The drawing under review shows one solid part. Ordinate dimensions are in mm from its lowest x, y, z. A direction names the side the tool comes from. Round coordinates to 2 decimals unless told otherwise and drop trailing zeros. Order: outer loops, then holes, each group sorted by start corner. A loop starts at its lowest first (then second) coordinate and runs counter-clockwise, first axis right, second up. Notation, with made-up numbers: M -14.5,30 L 40.5,30 A21 ccw 40.5,52 Z; hole C 17.5,59 d11. An arc over 180 degrees is marked long. Answer as a JSON object with one key per item and string values.
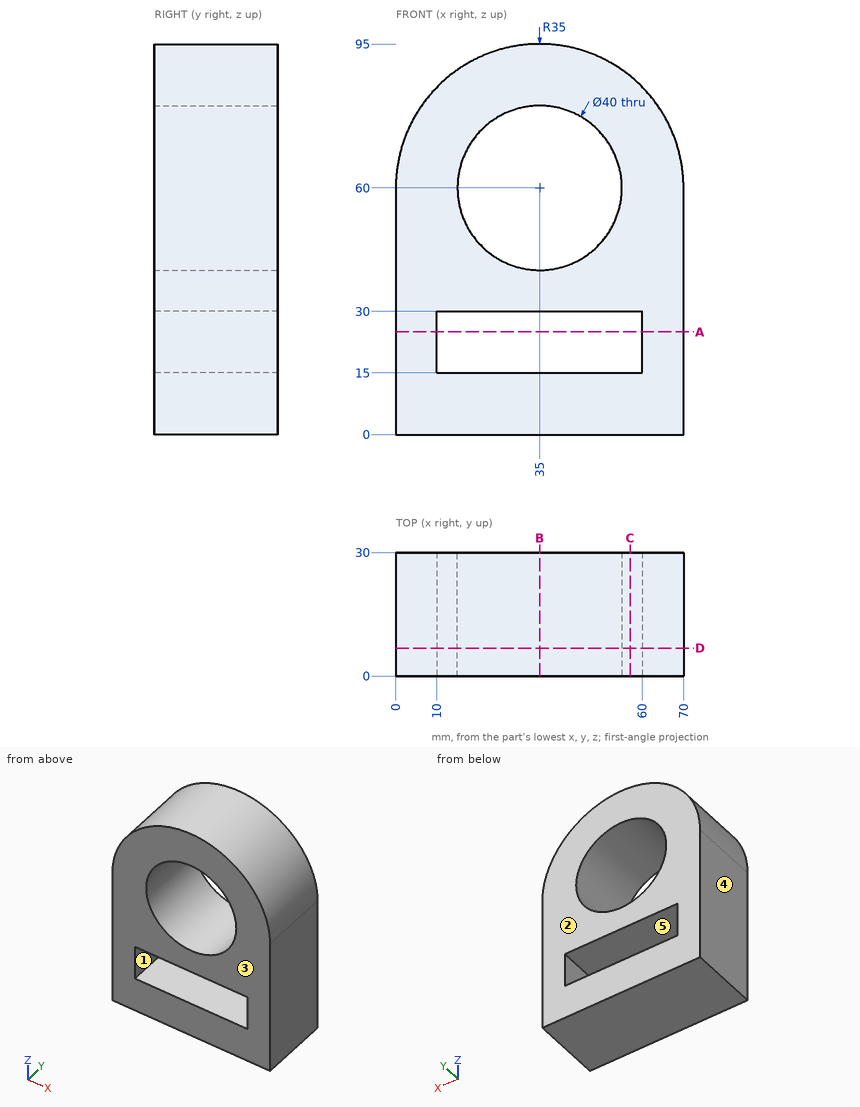
1) For L1, parallel to Z at x = 35, y = 22; L2, parallel to X at y = 21, z = 19; L3, parallel to Z at x = 33.5, y = 16.25, list the stretches that pass through material, from the lowest coordinate up.
Geometry check:
{"L1": "z = 0 to 15, 30 to 40, 80 to 95", "L2": "x = 0 to 10, 60 to 70", "L3": "z = 0 to 15, 30 to 40.06, 79.94 to 94.97"}
2) Insertion check: P1, Ø4, axis at y = 16.5, z = 65.5, coming from the +X side; P2, Ø6, axis at y = 10.5, z = 80.5, coming from the +X side; P3, Ø9, axis at x = 45, y = 22.5, coming from the +Z side. Each pin has a flat end and moves straight along its axis. Give the tip position at first contact, or say it passes through.
Geometry check:
{"P1": "stops at x = 69.82", "P2": "stops at x = 65.31", "P3": "stops at z = 94.57"}
3) Add section C-C on x = 57. State the section outline as (y, z) points.
Geometry check:
{"outline": "M 0,0 L 30,0 L 30,15 L 0,15 Z; M 0,30 L 30,30 L 30,87.22 L 0,87.22 Z"}
4) Machinability: for the marked faces 1 and 2, which of the approach directions +Z, -Z, +X, -X, +Y, -Y give a long, thin tool a straight path to every point of the face, cutting with its end or side? Answer none if there is none.
Geometry check:
{"face 1": "+Y, -Y", "face 2": "+Z, -Z, +X, -X, +Y"}
5) Add section B-B on x = 35. State the section outline as (y, z) points, and give its area (3 significant figures).
Geometry check:
{"outline": "M 0,0 L 30,0 L 30,15 L 0,15 Z; M 0,30 L 30,30 L 30,40 L 0,40 Z; M 0,80 L 30,80 L 30,95 L 0,95 Z", "area": "1,200 mm²"}
6) Add section A-A on z = 25. State the section outline as (x, y) points.
Geometry check:
{"outline": "M 0,0 L 10,0 L 10,30 L 0,30 Z; M 60,0 L 70,0 L 70,30 L 60,30 Z"}
7) Mouldability with a two-part tool opening along X and no side actions: class the marked faces 3, 4 and 5 as +X half, -X half, draft (parallel to the pull), parting line (faces both ways), or undercut.
Geometry check:
{"face 3": "draft", "face 4": "-X half", "face 5": "undercut"}
8) Add section D-D on y = 6.75. State the section outline as (x, z) points.
Geometry check:
{"outline": "M 0,0 L 70,0 L 70,60 A35 ccw 0,60 Z; hole M 10,15 L 60,15 L 60,30 L 10,30 Z; hole C 35,60 d40"}
